The model under review builds one solid part; all positions refer to its coordinate system, in mm. Face numbers are marked on the shaded views. A direction names the side the tool comes from. Coordinates: 2 decimals unless noted, no trailing zeros. Order: outer loops, then holes, each group sorted by start corner. A loop starts at its lowest first (then second) coordinate and runs counter-clockwise, first axis right, second up. Notation, with made-up numbers: (53.25, 42) -> (107.25, 42) arc R31 cw to (107.25, 80) -> close; hole circle Ø9 at (-24, 62.25). An arc over 180 degrees is marked (long way). Put each result on its own line as item: value.
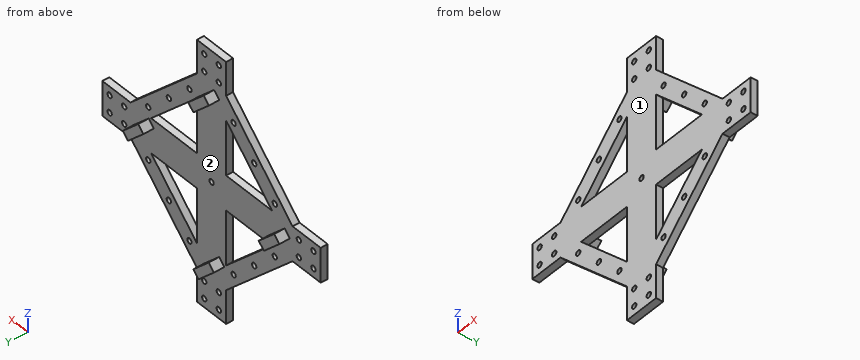
from build123d import *

# Parameters (mm, degrees)
SKETCH1_R             = 1.5
BASE_DEPTH            = 4
BATTERYCLIP_DEPTH     = 6
F_3_0MM_DOWEL_HOLE2_D = 3
CIRPATTERN2_COUNT     = 4


with BuildPart() as part:
    # Sketch1 → Base (new body)
    with BuildSketch(Plane(origin=(0, 0, 0), x_dir=(1, 0, 0), z_dir=(0, 1, 0))):
        Polygon((85, 85), (65.656854249, 85), (20, 130.656854249), (20, 150), (0, 150), (0, 130.656854249), (-45.656854249, 85), (-65, 85), (-65, 65), (-45.656854249, 65), (0, 19.343145751), (0, 0), (20, 0), (20, 19.343145751), (65.656854249, 65), (85, 65), align=None)
        Polygon((51.514718626, 85), (20, 85), (20, 116.514718626), align=None, mode=Mode.SUBTRACT)
        Polygon((-31.514718626, 65), (0, 65), (0, 33.485281374), align=None, mode=Mode.SUBTRACT)
        Polygon((0, 116.514718626), (0, 85), (-31.514718626, 85), align=None, mode=Mode.SUBTRACT)
        Polygon((20, 33.485281374), (20, 65), (51.514718626, 65), align=None, mode=Mode.SUBTRACT)
        with Locations(Location((10, 75, 0), (0, 0, 270))):
            Circle(SKETCH1_R, mode=Mode.SUBTRACT)
    extrude(amount=BASE_DEPTH)

    # Sketch2 → BatteryClip (add)
    with BuildSketch(Plane(origin=(0, 4, 0), x_dir=(1, 0, 0), z_dir=(0, 1, 0))):
        Polygon((15.303300859, 35.402020254), (4.696699141, 24.795418536), (8.232233047, 21.25988463), (18.838834765, 31.866486348), align=None)
        Polygon((11.767766953, 128.74011537), (1.161165235, 118.133513652), (4.696699141, 114.597979746), (15.303300859, 125.204581464), align=None)
        Polygon((49.597979746, 69.696699141), (60.204581464, 80.303300859), (63.74011537, 76.767766953), (53.133513652, 66.161165235), align=None)
        Polygon((-43.74011537, 73.232233047), (-33.133513652, 83.838834765), (-29.597979746, 80.303300859), (-40.204581464, 69.696699141), align=None)
    extrude(amount=BATTERYCLIP_DEPTH)

    # 3.0mm Dowel Hole2 (through all)
    with Locations(Plane(origin=(5, 4, -5), x_dir=(0, 0, 1), z_dir=(0, 1, 0))):
        with Locations((0, 0), (-10, 0), (-10, 10), (0, 10), (-26.564971157, -10.150757595), (-40.707106781, -24.292893219), (-54.849242405, -38.435028843)):
            f_3_0mm_dowel_hole2 = Hole(F_3_0MM_DOWEL_HOLE2_D / 2)

    # CirPattern2: 3.0mm Dowel Hole2 ×4 about axis
    cirpattern2_axis = Axis((10, 0, -75), (0, 1, 0))
    for i in range(1, CIRPATTERN2_COUNT):
        add(f_3_0mm_dowel_hole2.rotate(cirpattern2_axis, i * 360 / CIRPATTERN2_COUNT), mode=Mode.SUBTRACT)


solid = part.part
Item 1: Consider section B-B on z = -42. Write out the cut boundary in (x, y).
Answers below:
outline: (-22.66, 0) -> (-8.51, 0) -> (-8.51, 4) -> (-22.66, 4) -> close; (0, 0) -> (20, 0) -> (20, 4) -> (0, 4) -> close; (28.51, 0) -> (42.66, 0) -> (42.66, 4) -> (28.51, 4) -> close
Item 2: For pin 1 Ø5 at (x, y) = (-30.5, 4.5) entering from +Z; pin 2 Ø6 at (y, z) = (4.5, -44) entering from +X; pin 3 Ø5 at (x, z) = (5, -135) entering from -Y; pin 4 Ø3.5 at (x, z) = (-60, -70) entering from +Y, all flat-tipped, find the tip position at first contact; note any pin that passes through.
Answers below:
pin 1: z = -47.39
pin 2: x = 47.61
pin 3: y = 0
pin 4: y = 4
Item 3: For the marked faces 1 and 2, list the 3-axis set-ups (+Z, -Z, +X, -X, +Y, -Y) from which the entire face can be reached by the end or side of a thin tool; tool diameter is ignored.
Answers below:
face 1: +Z, -Z, +X, -X, -Y
face 2: +Y
Item 4: For line 1 (Z direction, x = 80, y = 1.75); line 2 (Z direction, x = -7.5, y = 1.75); line 3 (X direction, y = 1.25, z = -49), list the stretches that pass through material, from the lowest coordinate up. Write a range as from..to.
Answers below:
line 1: -85..-81.5, -78.5..-71.5, -68.5..-65
line 2: -123.16..-109.01, -85..-65, -40.99..-26.84
line 3: -29.66..-15.51, 0..20, 35.51..49.66
Item 5: Consider section A-A on y = 8. Write out the cut boundary in (x, z).
Answers below:
outline: (-43.74, -73.23) -> (-33.13, -83.84) -> (-29.6, -80.3) -> (-40.2, -69.7) -> close; (1.16, -118.13) -> (11.77, -128.74) -> (15.3, -125.2) -> (4.7, -114.6) -> close; (4.7, -24.8) -> (15.3, -35.4) -> (18.84, -31.87) -> (8.23, -21.26) -> close; (49.6, -69.7) -> (60.2, -80.3) -> (63.74, -76.77) -> (53.13, -66.16) -> close
